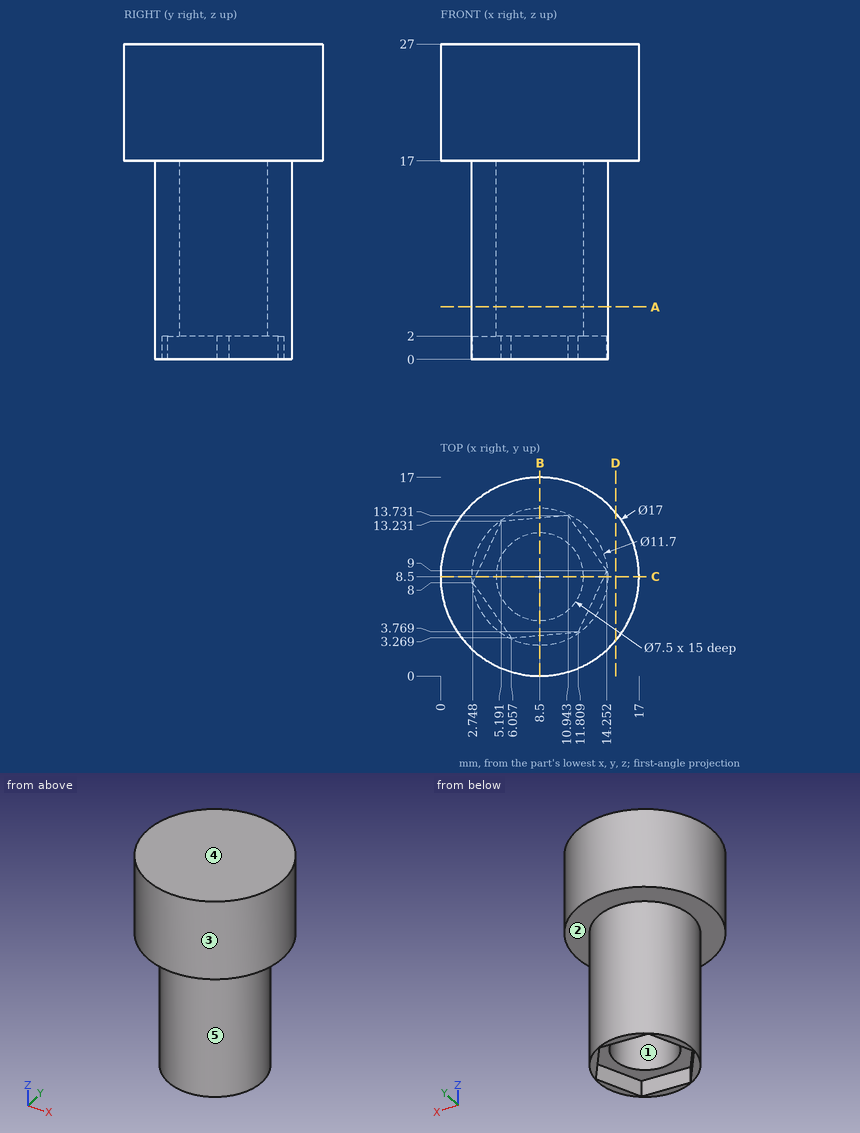
Check sheet for the drawn part. Datum: minimum x, y, z corner. Units: mm. A direction names the side the tool comes from. Coordinates: 2 decimals unless noted, no trailing zeros. Write each loop counter-clockwise with the first axis right and the second up, starting at its lowest first coordinate (ties: lowest second). Pieces come first, ordered by that corner, then holes. Notation, with made-up numbers: M 64,-15 L 96,-15 A18 cw 96,20 Z; hole C 67,32 d8. An arc over 180 degrees is marked long. Use a Markdown table: item, result.
Q1. Set-up check for the marked faces 4 and 5: record each of +Z, -Z, +X, -X, +Y, -Y from which the full face is reachable in a straight line by a thin tool's end or side.
Reply:
| item | result |
|---|---|
| face 4 | +Z, +X, -X, +Y, -Y |
| face 5 | -Z |
Q2. Sectioned sample at C-C, the plane y = 8.5. Record the boundary of the cut face in (x, z), plus the area to 3 significant figures.
Reply:
| item | result |
|---|---|
| outline | M 0,17 L 2.65,17 L 2.65,0 L 2.98,0 L 2.98,2 L 4.75,2 L 4.75,17 L 12.25,17 L 12.25,2 L 14.02,2 L 14.02,0 L 14.35,0 L 14.35,17 L 17,17 L 17,27 L 0,27 Z |
| area | 234 mm² |
Q3. Sectioned sample at A-A, the plane z = 4.5. Record the boundary of the cut face in (x, y).
Reply:
| item | result |
|---|---|
| outline | C 8.5,8.5 d11.7; hole C 8.5,8.5 d7.5 |
Q4. Sectioned sample at D-D, the plane x = 15. Record the boundary of the cut face in (y, z), plus the area to 3 significant figures.
Reply:
| item | result |
|---|---|
| outline | M 3.02,17 L 13.98,17 L 13.98,27 L 3.02,27 Z |
| area | 110 mm² |
Q5. Draft check along Y on the marked faces 1, 2 and 3. Enter one of: +Y half, -Y half, draft (parallel to the pull), parting line (faces both ways), or undercut.
Reply:
| item | result |
|---|---|
| face 1 | undercut |
| face 2 | draft |
| face 3 | parting line |
Q6. Go/stop test with flat-tipped pins: P1, Ø6, axis at x = 3.5, z = 6, coming from the +Y side; P2, Ø5, axis at y = 5, z = 3.5, coming from the -X side; P3, Ø6, axis at x = 2.5, z = 21, coming from the -Y side. Record where each tip stops, or that it passes through.
Reply:
| item | result |
|---|---|
| P1 | stops at y = 14 |
| P2 | stops at x = 2.74 |
| P3 | stops at y = 0.55 |
Q7. Sectioned sample at B-B, the plane x = 8.5. Record the boundary of the cut face in (y, z).
Reply:
| item | result |
|---|---|
| outline | M 0,17 L 2.65,17 L 2.65,0 L 3.48,0 L 3.48,2 L 4.75,2 L 4.75,17 L 12.25,17 L 12.25,2 L 13.52,2 L 13.52,0 L 14.35,0 L 14.35,17 L 17,17 L 17,27 L 0,27 Z |
Q8. Thickness scan on line 1 (Y direction, x = 8.5, z = 10.5); line 2 (Z direction, x = 2, y = 10.75); line 3 (X direction, y = 6.5, z = 8.5). Record the ranges inside material, lowest first.
Reply:
| item | result |
|---|---|
| line 1 | y = 2.65 to 4.75, 12.25 to 14.35 |
| line 2 | z = 17 to 27 |
| line 3 | x = 3 to 5.33, 11.67 to 14 |
